CAD build for the part. Positions are in the model's coordinates, mm. A direction names the side the tool comes from. Coordinates: 2 decimals unless noted, no trailing zeros. Loops run counter-clockwise (first coordinate to the right, second up) from the corner with the lowest first, then second, coordinate; pieces in that order, holes last.
1) Pin check, flat tips, straight feed: pin 1 Ø6 at (y, z) = (-5.5, -8) entering from +X; pin 2 Ø5 at (y, z) = (1.5, -4.5) entering from +X; pin 3 Ø12 at (x, z) = (-5, -8.5) entering from -Y; pin 4 Ø2 at (x, y) = (3.5, -9.5) entering from +Z. Stop position of each tip, or through.
2) Wall check: line 1 along Z through (x, y) = (-0.25, -11.25); line 2 along Y through (x, z) = (6.25, 9.75). Give the ranges that are in metal, low to high.
3) Which spindle directions (+Z, -Z, +X, -X, +Y, -Y) get a long thin tool onto all of the face, cutting with end or side? Do faces 1 (the cylindrical face through (-6.834, -7.395, 1.517)), 2 (the flat face through (0, 7.55, 0)). Say none if no direction does.
4) Saw through at B-B, the plane y = 6. Write the cut outline in (x, z).
5) Saw through at D-D, the plane y = -7.25. Write the cut outline in (x, z).
6) Saw through at A-A, the plane x = 0. Write the cut outline in (y, z).
7) Saw through at C-C, the plane z = 8.5. Write the cut outline in (x, y), and give its area (3 significant figures).
```python
from build123d import *

# Parameters (mm, degrees)
BOSS_EXTRUDE1_DEPTH = 7.55
SKETCH2_R           = 7
BOSS_EXTRUDE2_DEPTH = 16
CHAMFER1_SIZE       = 1


with BuildPart() as part:
    # Sketch1 → Boss-Extrude1 (new body)
    with BuildSketch(Plane(origin=(0, 0, 0), x_dir=(1, 0, 0), z_dir=(0, 1, 0))):
        Polygon((-12.124355653, 0), (-6.062177826, -10.5), (6.062177826, -10.5), (12.124355653, 0), (6.062177826, 10.5), (-6.062177826, 10.5), align=None)
    extrude(amount=BOSS_EXTRUDE1_DEPTH)

    # Sketch2 → Boss-Extrude2 (add)
    with BuildSketch(Plane.XZ):
        with Locations(Location((0, 0, 0), (0, 0, 270))):
            Circle(SKETCH2_R)
    extrude(amount=BOSS_EXTRUDE2_DEPTH)

    # Chamfer1
    chamfer1_edges = [part.edges().sort_by_distance(p)[0] for p in [
        (0, -16, 7),
    ]]
    chamfer(chamfer1_edges, length=CHAMFER1_SIZE)


solid = part.part
```
Data:
1. pin 1: stops at x = 4.9
1. pin 2: stops at x = 10.97
1. pin 3: stops at y = -16
1. pin 4: stops at z = 6.54
2. line 1: z = -7 to 7
2. line 2: y = 0 to 7.55
3. face 1: -Y
3. face 2: +Z, -Z, +X, -X, +Y
4. outline: (-12.12, 0) - (-6.06, -10.5) - (6.06, -10.5) - (12.12, 0) - (6.06, 10.5) - (-6.06, 10.5) - close
5. outline: circle Ø14 at (0, 0)
6. outline: (-16, -6) - (-15, -7) - (0, -7) - (0, -10.5) - (7.55, -10.5) - (7.55, 10.5) - (0, 10.5) - (0, 7) - (-15, 7) - (-16, 6) - close
7. outline: (-7.22, 0) - (7.22, 0) - (7.22, 7.55) - (-7.22, 7.55) - close
7. area: 109 mm2
